```python
from build123d import *

# Parameters (mm, degrees)
SKETCH_1_R          = 215
EXTRUDE_1_DEPTH     = 0.2
CUT_EXTRUDE_2_REACH = 306.056
SKETCH_4_R          = 3
SKETCH_4_W          = 22
SKETCH_4_H          = 22


with BuildPart() as part:
    # Эскиз1 → Бобышка-Вытянуть1 (new body)
    with BuildSketch(Plane(origin=(0, 0, 0), x_dir=(1, 0, 0), z_dir=(0, 1, 0))):
        with Locations(Location((0, 0, 0), (0, 0, 270))):
            Circle(SKETCH_1_R)
    extrude(amount=EXTRUDE_1_DEPTH)

    # Эскиз4 → Вырез-Вытянуть2 (cut, up to next)
    with BuildSketch(Plane(origin=(0, 0.2, 0), x_dir=(1, 0, 0), z_dir=(0, 1, 0)), mode=Mode.PRIVATE) as cut_extrude_2_sk1:
        with Locations(Location((0, 41, 0), (0, 0, 270))):
            Circle(SKETCH_4_R)
    cut_extrude_2_tool1 = extrude(cut_extrude_2_sk1.sketch, amount=-CUT_EXTRUDE_2_REACH, mode=Mode.PRIVATE) & part.part
    # Эскиз4 → Вырез-Вытянуть2 (cut, up to next)
    with BuildSketch(Plane(origin=(0, 0.2, 0), x_dir=(1, 0, 0), z_dir=(0, 1, 0)), mode=Mode.PRIVATE) as cut_extrude_2_sk2:
        with Locations(Location((41, 0, 0), (0, 0, 270))):
            Circle(SKETCH_4_R)
    cut_extrude_2_tool2 = extrude(cut_extrude_2_sk2.sketch, amount=-CUT_EXTRUDE_2_REACH, mode=Mode.PRIVATE) & part.part
    # Эскиз4 → Вырез-Вытянуть2 (cut, up to next)
    with BuildSketch(Plane(origin=(0, 0.2, 0), x_dir=(1, 0, 0), z_dir=(0, 1, 0)), mode=Mode.PRIVATE) as cut_extrude_2_sk3:
        with Locations(Location((0, -41, 0), (0, 0, 270))):
            Circle(SKETCH_4_R)
    cut_extrude_2_tool3 = extrude(cut_extrude_2_sk3.sketch, amount=-CUT_EXTRUDE_2_REACH, mode=Mode.PRIVATE) & part.part
    # Эскиз4 → Вырез-Вытянуть2 (cut, up to next)
    with BuildSketch(Plane(origin=(0, 0.2, 0), x_dir=(1, 0, 0), z_dir=(0, 1, 0)), mode=Mode.PRIVATE) as cut_extrude_2_sk4:
        with Locations(Location((-41, 0, 0), (0, 0, 270))):
            Circle(SKETCH_4_R)
    cut_extrude_2_tool4 = extrude(cut_extrude_2_sk4.sketch, amount=-CUT_EXTRUDE_2_REACH, mode=Mode.PRIVATE) & part.part
    # Эскиз4 → Вырез-Вытянуть2 (cut, up to next)
    with BuildSketch(Plane(origin=(0, 0.2, 0), x_dir=(1, 0, 0), z_dir=(0, 1, 0)), mode=Mode.PRIVATE) as cut_extrude_2_sk5:
        Rectangle(SKETCH_4_W, SKETCH_4_H)
    cut_extrude_2_tool5 = extrude(cut_extrude_2_sk5.sketch, amount=-CUT_EXTRUDE_2_REACH, mode=Mode.PRIVATE) & part.part
    add(cut_extrude_2_tool1.solids().sort_by_distance((0, 0.2, -41))[0], mode=Mode.SUBTRACT)
    add(cut_extrude_2_tool2.solids().sort_by_distance((41, 0.2, 0))[0], mode=Mode.SUBTRACT)
    add(cut_extrude_2_tool3.solids().sort_by_distance((0, 0.2, 41))[0], mode=Mode.SUBTRACT)
    add(cut_extrude_2_tool4.solids().sort_by_distance((-41, 0.2, 0))[0], mode=Mode.SUBTRACT)
    add(cut_extrude_2_tool5.solids().sort_by_distance((0, 0.2, 0))[0], mode=Mode.SUBTRACT)


solid = part.part
```
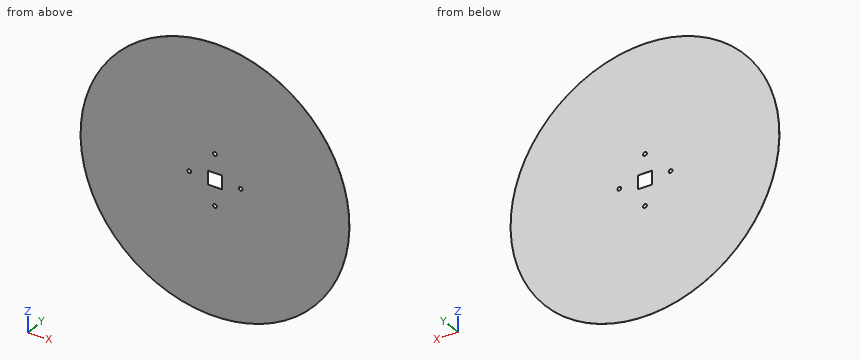
Check sheet for the modelled part. Datum: model origin and axes. Units: mm. Round coordinates to 2 decimals unless told otherwise and drop trailing zeros. Order: outer loops, then holes, each group sorted by start corner. A loop starts at its lowest first (then second) coordinate and runs counter-clockwise, first axis right, second up. Notation, with made-up numbers: (51.5, 30) - (67.5, 30) arc R15 cw to (67.5, 48) - close; hole circle Ø5 at (-15.75, 87.5). An arc over 180 degrees is marked (long way). Answer as CSV lines item,"result". Start each with the question number.
1) Scan lines: probe 1 along X at (y, z) = (0.1, -0.5); probe 2 along X at (y, z) = (0.15, 41); probe 3 along Z at (x, y) = (161, 0.1). Record each from-to range of solid material in increasing order.
2) Depth check by flat-ended pin: pin 1 (5.5 mm diameter, centred on x = 0, z = -41, fed in from -Y). Enter the tip coordinate at first touch or a pass-through.
3) Section check C-C (z = -175.5). Record the cut outline in (x, y), then the cut area to 3 significant figures.
4) Section check A-A (y = 0.1). Record the cut outline in (x, z), then the cut area to 3 significant figures.
5) Section check B-B (x = 139). Record the cut outline in (y, z), then the cut area to 3 significant figures.
Determined:
1,probe 1,"-215 to -43.96, -38.04 to -11, 11 to 38.04, 43.96 to 215"
1,probe 2,"-211.05 to -3, 3 to 211.05"
1,probe 3,"-142.49 to 142.49"
2,pin 1,"through"
3,outline,"(-124.2, 0) - (124.2, 0) - (124.2, 0.2) - (-124.2, 0.2) - close"
3,area,"49.7 mm^2"
4,outline,"circle Ø430 at (0, 0); hole circle Ø6 at (-41, 0); hole (-11, -11) - (11, -11) - (11, 11) - (-11, 11) - close; hole circle Ø6 at (0, -41); hole circle Ø6 at (0, 41); hole circle Ø6 at (41, 0)"
4,area,"145,000 mm^2"
5,outline,"(0, -164.02) - (0.2, -164.02) - (0.2, 164.02) - (0, 164.02) - close"
5,area,"65.6 mm^2"
